Here's the drawing with two shaded views (mm, measured from the low corner). I have some questions. Round coordinates to 2 decimals unless told otherwise and drop trailing zeros. Loops run counter-clockwise (first coordinate to the right, second up) from the corner with the lowest first, then second, coordinate; pieces in that order, holes last. Notation, with made-up numbers: M 52.5,70.5 L 85.5,70.5 A25 ccw 85.5,88.5 Z; hole C 88,75 d2. An arc over 180 degrees is marked long. One line per item, written item: value. Start each with the question number.
Q1. Imagine slicing it at D-D (y = 35). Please give me the cut outline in (x, z).
Q2. Imagine slicing it at A-A (x = 0.7). Please give me the cut outline in (y, z).
Q3. Imagine slicing it at B-B (y = 20). Please give me the cut outline in (x, z), then the cut area to 3 significant figures.
Q4. Please list where these lines run through material, in increasing order: line 1 along Y through (x, z) = (0.75, 20); line 2 along Y through (x, z) = (2.7, 21.5); line 3 along Y through (x, z) = (0.7, 27.24).
Q5. I'm going to push flat-ended pins straight in: pin 1 Ø1.5 at (x, y) = (1.5, 21) entering from -Z; pin 2 Ø1.5 at (x, z) = (1.5, 9) entering from +Y; pin 3 Ø1.6 at (y, z) = (20, 27.24) entering from -X; pin 4 Ø0.9 at (x, y) = (1, 14.5) entering from +Z. Where does each tip first touch, or does it pass through?
Q6. Imagine slicing it at C-C (z = 12.76). Please give me the cut outline in (x, y).
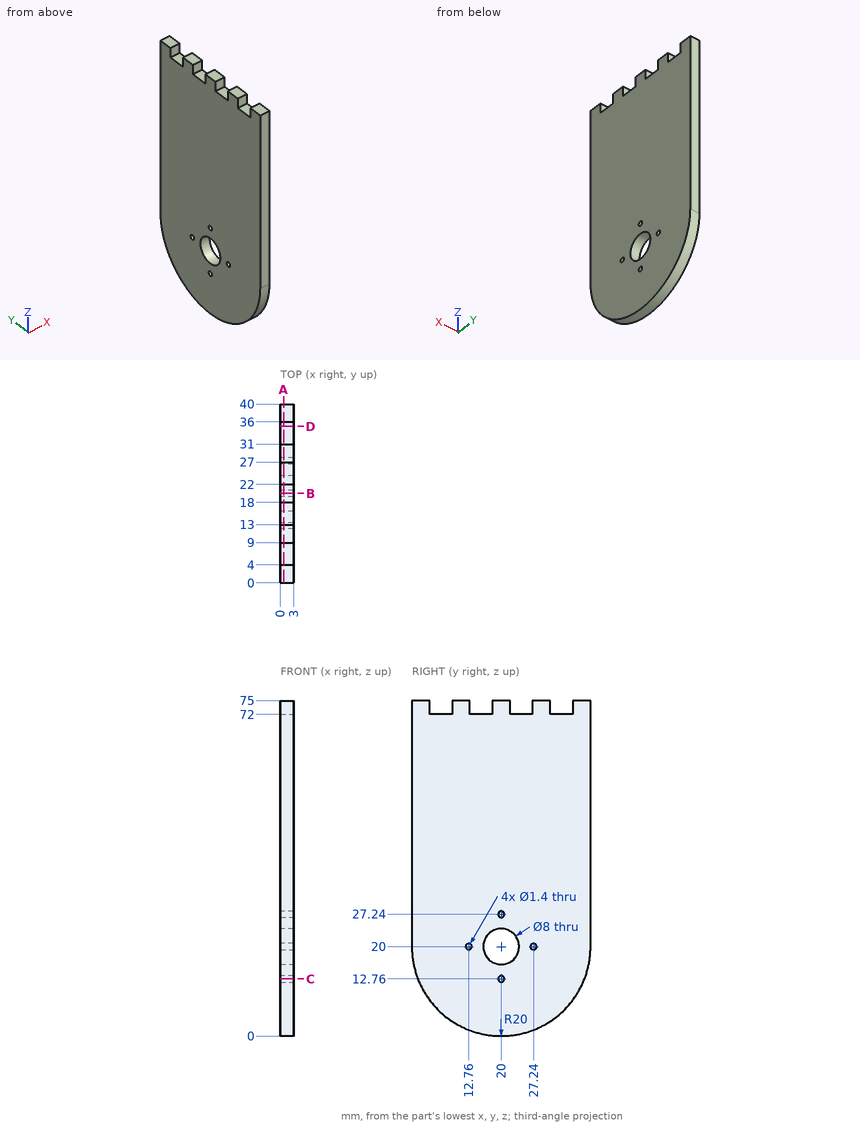
Report:
1. outline: M 0,6.77 L 3,6.77 L 3,72 L 0,72 Z
2. outline: M 0,20 A20 ccw 40,20 L 40,75 L 36,75 L 36,72 L 31,72 L 31,75 L 27,75 L 27,72 L 22,72 L 22,75 L 18,75 L 18,72 L 13,72 L 13,75 L 9,75 L 9,72 L 4,72 L 4,75 L 0,75 Z; hole C 12.76,20 d1.4; hole C 20,20 d8; hole C 20,12.76 d1.4; hole C 20,27.24 d1.4; hole C 27.24,20 d1.4
3. outline: M 0,0 L 3,0 L 3,12.06 L 0,12.06 Z; M 0,13.46 L 3,13.46 L 3,16 L 0,16 Z; M 0,24 L 3,24 L 3,26.54 L 0,26.54 Z; M 0,27.94 L 3,27.94 L 3,75 L 0,75 Z
3. area: 193 mm²
4. line 1: y = 0 to 12.06, 13.46 to 16, 24 to 26.54, 27.94 to 40
4. line 2: y = 0 to 16.29, 23.71 to 40
4. line 3: y = 0 to 19.3, 20.7 to 40
5. pin 1: stops at z = 0
5. pin 2: stops at y = 37.17
5. pin 3: stops at x = 0
5. pin 4: stops at z = 72
6. outline: M 0,1.36 L 3,1.36 L 3,19.3 L 0,19.3 Z; M 0,20.7 L 3,20.7 L 3,38.64 L 0,38.64 Z
